```python
from build123d import *

# Parameters (mm, degrees)
SKETCH1_R               = 75.946
BOSS_EXTRUDE1_DEPTH     = 10.16
SKETCH7_R               = 74.295
BOSS_EXTRUDE2_DEPTH     = 1.27
SKETCH6_R               = 3.183478234
SKETCH6_R_2             = 3.2
SKETCH6_R_3             = 3.175
CUT_EXTRUDE5_DEPTH      = 2.27
CUT_EXTRUDE5_DEPTH_BACK = 11.16
SKETCH9_R               = 57.4675
CUT_EXTRUDE7_DEPTH      = 12.43


with BuildPart() as part:
    # Sketch1 → Boss-Extrude1 (new body)
    with BuildSketch(Plane(origin=(0, 0, 0), x_dir=(1, 0, 0), z_dir=(0, 1, 0))):
        Circle(SKETCH1_R)
    extrude(amount=BOSS_EXTRUDE1_DEPTH)

    # Sketch7 → Boss-Extrude2 (add)
    with BuildSketch(Plane(origin=(0, 10.16, 0), x_dir=(1, 0, 0), z_dir=(0, 1, 0))):
        Circle(SKETCH7_R)
    extrude(amount=BOSS_EXTRUDE2_DEPTH)

    # Sketch6 → Cut-Extrude5 (cut, two sides)
    with BuildSketch(Plane(origin=(0, 10.16, 0), x_dir=(1, 0, 0), z_dir=(0, 1, 0))) as cut_extrude5_sk:
        with Locations((-64.77, 0)):
            Circle(SKETCH6_R)
        with Locations((-32.260478415, 56.164173923)):
            Circle(SKETCH6_R_2)
        with Locations((-32.385, -56.092465403)):
            Circle(SKETCH6_R_3)
        with Locations((32.385, -56.092465403)):
            Circle(SKETCH6_R_3)
        with Locations((64.77, 0)):
            Circle(SKETCH6_R)
        with Locations((32.260478415, 56.164173923)):
            Circle(SKETCH6_R_2)
    extrude(amount=CUT_EXTRUDE5_DEPTH, mode=Mode.SUBTRACT)
    extrude(cut_extrude5_sk.sketch, amount=-CUT_EXTRUDE5_DEPTH_BACK, mode=Mode.SUBTRACT)

    # Sketch9 → Cut-Extrude7 (cut, through all)
    with BuildSketch(Plane(origin=(0, 11.43, 0), x_dir=(1, 0, 0), z_dir=(0, 1, 0))):
        Circle(SKETCH9_R)
    extrude(amount=-CUT_EXTRUDE7_DEPTH, mode=Mode.SUBTRACT)


solid = part.part
```
The model under review builds one solid part; all positions refer to its coordinate system, in mm. A direction names the side the tool comes from. Round coordinates to 2 decimals unless told otherwise and drop trailing zeros. Write each loop counter-clockwise with the first axis right and the second up, starting at its lowest first coordinate (ties: lowest second). Pieces come first, ordered by that corner, then holes.
(1) We need section B-B on z = 0. Give the boundary of the cut face in (x, y) (1 decimal).
(2) We need section C-C on z = 41.5. Give the boundary of the cut face in (x, y).
(3) We need section A-A on x = 0. Give the boundary of the cut face in (y, z) (1 decimal).
(4) We need section D-D on y = 5.25. Give the number of separate pieces and of enclosed holes in the cut face, and give its area (3 significant figures).
(5) Wall thickness on L1, parallel to X at y = 3.25, z = -0.5; L2, parallel to X at y = 9, z = 0; L3, parallel to Z at x = 33, y = 11: over which ranges is each line inside the solid? List them lowest first.
(6) Mouldability with a two-part tool opening along X and no side actions: class faces 3 (the cylindrical face through (31.844, 5.795, -59.337)), 4 (the flat face through (-57, 0, 11)), 5 (the cylindrical face through (-58.958, 10.786, 45.207)) as +X half, -X half, draft (parallel to the pull), parting line (faces both ways), or undercut.
(7) Insertion check: pin 1 (8 mm diameter, centred on x = 17, z = -48.5, fed in from +Y); pin 2 (2 mm diameter, centred on y = 4, z = 27, fed in from +X); pin 3 (4 mm diameter, centred on x = 25.5, y = 2, fed in from +Z); pin 4 (2 mm diameter, centred on x = -46.5, y = 9.5, fed in from -Z). Each pin has a flat end and moves straight along its axis. Give the tip position at first contact, or say it passes through.
(8) Machinability: for faces 1 (the flat face through (56, 10.16, 50)), 2 (the cylindrical face through (-32.677, 5.795, -59.337)), which of the approach directions +Z, -Z, +X, -X, +Y, -Y give a long, thin tool a straight path to every point of the face, cutting with its end or side? Answer none if there is none.
Findings below:
1. outline: (-75.9, 0) - (-68, 0) - (-68, 11.4) - (-74.3, 11.4) - (-74.3, 10.2) - (-75.9, 10.2) - close; (-61.6, 0) - (-57.5, 0) - (-57.5, 11.4) - (-61.6, 11.4) - close; (57.5, 0) - (61.6, 0) - (61.6, 11.4) - (57.5, 11.4) - close; (68, 0) - (75.9, 0) - (75.9, 10.2) - (74.3, 10.2) - (74.3, 11.4) - (68, 11.4) - close
2. outline: (-63.6, 0) - (-39.75, 0) - (-39.75, 11.43) - (-61.62, 11.43) - (-61.62, 10.16) - (-63.6, 10.16) - close; (39.75, 0) - (63.6, 0) - (63.6, 10.16) - (61.62, 10.16) - (61.62, 11.43) - (39.75, 11.43) - close
3. outline: (0, -75.9) - (10.2, -75.9) - (10.2, -74.3) - (11.4, -74.3) - (11.4, -57.5) - (0, -57.5) - close; (0, 57.5) - (11.4, 57.5) - (11.4, 74.3) - (10.2, 74.3) - (10.2, 75.9) - (0, 75.9) - close
4. separate pieces: 1
4. enclosed holes: 7
4. area: 7,550 mm2
5. L1: x = -75.94 to -67.91, -61.63 to -57.47, 57.47 to 61.63, 67.91 to 75.94
5. L2: x = -75.95 to -67.95, -61.59 to -57.47, 57.47 to 61.59, 67.95 to 75.95
5. L3: z = -66.56 to -59.28, -53.05 to -47.05, 47.05 to 52.98, 59.21 to 66.56
6. face 3: undercut
6. face 4: draft
6. face 5: parting line
7. pin 1: passes through
7. pin 2: stops at x = 71.36
7. pin 3: stops at z = 72.22
7. pin 4: stops at z = -60.81
8. face 1: +Y
8. face 2: +Y, -Y
